Design review of the part built by this model. Coordinates are the model's own, in mm. Give positions to 0.01 mm unless a question says otherwise; leave off trailing zeros. Order: outer loops, then holes, each group sorted by start corner. A loop starts at its lowest first (then second) coordinate and runs counter-clockwise, first axis right, second up. Notation, with made-up numbers: M 15.25,65 L 25.25,65 A25 ccw 25.25,94 Z; hole C 1.25,-19 d3. An arc over 180 degrees is marked long. Answer as a JSON object with one key per item and string values.
Autodesk Inventor part; units mm, degrees
ref_plane "Work Plane1" through (381, 0, 0) normal (1, 0, 0) x (0, 1, 0)
ref_plane "XZ Plane" through (0, 0, 0) normal (0, 1, 0) x (-1, 0, 0)
ref_plane "XY Plane" through (0, 0, 0) normal (0, 0, 1) x (1, 0, 0)
sketch "Sketch1" plane through (0, 0, 0) normal (0, 0, 1) x (1, 0, 0)
  circle A0 centre (0, 0) radius 12.7
  dimension "d0" = 25.4
sketch "Sketch2" plane through (0, 0, 0) normal (1, 0, 0) x (0, 1, 0)
  line L0 (0, 88.9) -> (0, -88.9)
  line L1 (0, -88.9) -> (48.2558, -206.375)
  line L2 (0, 88.9) -> (48.2558, 206.375)
  line L3 (48.2558, -206.375) -> (232.1871, -206.375) construction
  point P0 (0, 0)
  dimension "d1" = 88.9
  dimension "d2" = 177.8
  dimension "d3" = 412.75
  dimension "d5" = 127
  dimension "d26" = 112.332
sweep "Sweep1" add profiles "Sketch1" path "Sketch2"
ref_plane "Work Plane1" through (381, 0, 0) normal (1, 0, 0) x (0, 1, 0)
sketch "Sketch3" plane through (0, 0, 0) normal (0, 0, 1) x (1, 0, 0)
  circle A0 centre (381, 0) radius 12.7
  point P0 (0, 0)
  dimension "d9" = 381
  dimension "d10" = 25.4
sketch "Sketch4" plane through (381, 0, 0) normal (1, 0, 0) x (0, 1, 0)
  line L0 (60.0033, 201.5494) -> (36.5083, 211.2006)
  line L1 (48.2558, 206.375) -> (0, 158.75)
  line L2 (0, 158.75) -> (0, -158.75)
  line L3 (0, -158.75) -> (48.2558, -206.375)
  line L4 (36.5083, -211.2006) -> (60.0033, -201.5494)
  point P0 (0, 0)
  point P1 (0, 0)
  dimension "d11" = 317.5
  dimension "d13" = 0
sweep "Sweep2" add profiles "Sketch3" path "Sketch4" path curves L3 L2 L1
sketch "Sketch5" plane through (0, 0, 0) normal (1, 0, 0) x (0, 1, 0)
  line L0 (39.3348, -215.4141) -> (57.1768, -197.3359)
  line L1 (36.5083, -211.2006) -> (60.0033, -201.5494)
  line L2 (57.1768, 197.3359) -> (39.3348, 215.4141)
  line L3 (60.0033, 201.5494) -> (36.5083, 211.2006)
  circle A0 centre (48.2558, 206.375) radius 14.351
  circle A1 centre (48.2558, -206.375) radius 14.351
  point P0 (0, 0)
  dimension "d16" = 28.702
extrude "Extrusion1" add sketch "Sketch5" along normal blind 635 and the other way blind 50.8
sketch "Sketch6" plane through (0, 0, 0) normal (1, 0, 0) x (0, 1, 0)
  circle A0 centre (48.2558, 206.375) radius 14.351
  circle A1 centre (48.2558, -206.375) radius 14.351
  circle A2 centre (48.2558, -206.375) radius 19.812
  circle A3 centre (48.2558, 206.375) radius 19.812
  point P0 (0, 0)
  dimension "d21" = 39.624
extrude "Extrusion2" add sketch "Sketch6" along normal mid plane 28.575 contours A0 | A1 | A2 | A3
sketch "Sketch7" plane through (-50.8, 48.2558, 206.375) normal (-1, 0, 0) x (0, 0, 1)
  circle A0 centre (-412.75, 0) radius 14.351
  circle A1 centre (0, 0) radius 14.351
  circle A2 centre (-412.75, 0) radius 19.812
  circle A3 centre (0, 0) radius 19.812
  point P0 (-206.375, -48.2558)
extrude "Extrusion3" add sketch "Sketch7" against normal blind 6.35 contours A0 | A1 | A2 | A3
properties part number "front bar" material "Aluminum 6061"
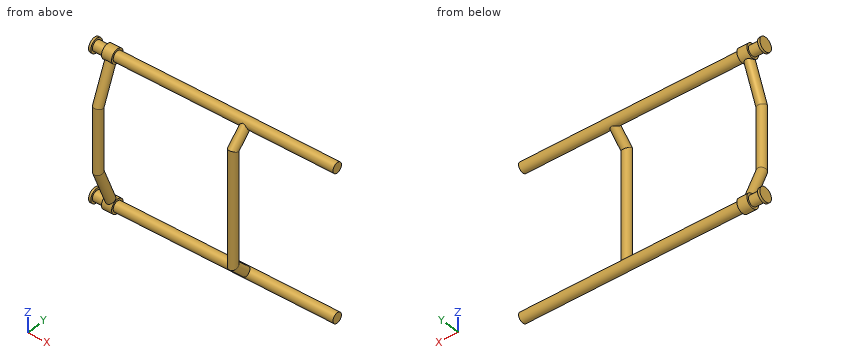
(1) We need section B-B (x = 0). Write out the cut boundary in (y, z) (3 decimals).
Checked values:
{"outline": "M -12.7,-91.407 L 30.73,-197.135 A19.812 ccw long 54.225,-187.484 L 12.7,-86.393 L 12.7,86.393 L 54.225,187.484 A19.812 ccw long 30.73,197.135 L -12.7,91.407 Z"}
(2) To check wall thickness, follow L1, parallel to X at y = 0, z = -35; L2, parallel to Z at x = 474, y = 61; L3, parallel to Y at x = 406, z = 205.5. State the ranges of each line that lie inside material, in increasing order. Write a range as from..to.
Checked values:
{"L1": "x = -12.7..12.7, 368.3..393.7", "L2": "z = -212.97..-199.78, 199.78..212.97", "L3": "y = 33.93..62.58"}
(3) We need section A-A (z = -21). Write out the cut boundary in (x, y), plus the area to 3 significant figures.
Checked values:
{"outline": "C 0,0 d25.4; C 381,0 d25.4", "area": "1,010 mm^2"}
(4) We need section C-C (x = 266). Write out the cut boundary in (y, z) (3 decimals).
Checked values:
{"outline": "C 48.256,-206.375 d28.702; C 48.256,206.375 d28.702"}
(5) Insertion check: pin 1 (2 mm diameter, centred on x = 377.5, y = 55, fed in from -Z); pin 2 (6 mm diameter, centred on x = 376, z = 59.5, fed in from -Y); pin 3 (2 mm diameter, centred on x = 372.5, y = 13, fed in from -Z). Each pin has a flat end and moves straight along its axis. Give the tip position at first contact, or say it passes through.
Checked values:
{"pin 1": "stops at z = -219.53", "pin 2": "stops at y = -12.54", "pin 3": "stops at z = -186.37"}
